Part model, mm, in its own coordinate system. Give positions to 0.01 mm unless a question says otherwise; leave off trailing zeros. Order: outer loops, then holes, each group sorted by start corner. A loop starts at its lowest first (then second) coordinate and runs counter-clockwise, first axis right, second up. Notation, with made-up numbers: M -7,-1 L 41,-1 A20 ccw 41,21 Z; hole C 74.5,-27.5 d11. An arc over 180 degrees is marked long. Return JSON: item names as keys, results as strings.
from build123d import *

# Parameters (mm, degrees)
SKETCH1_W                        = 2413
SKETCH1_H                        = 41.5544
BASE_FLANGE1_DEPTH               = 3.2639
SKETCH66_R                       = 38.1
BOSS_EXTRUDE1_DEPTH              = 3.2639
EDGE_FLANGE1_DEPTH               = 1129.41735
EDGE_FLANGE1_BEND_DEPTH          = 1066.86985
EDGE_FLANGE1_BEND_2_DEPTH        = 1066.86985
EDGE_FLANGE1_BEND_3_DEPTH        = 1129.41735
F_10_0_1935_DIAMETER_HOLE1_D     = 4.9149
F_10_0_1935_DIAMETER_HOLE1_DEPTH = 3.2649
LPATTERN1_COUNT                  = 6
LPATTERN1_PITCH                  = 215.265
F_10_0_1935_DIAMETER_HOLE2_D     = 4.9149
LPATTERN2_START                  = 22.0472
LPATTERN2_OUTLINE_R              = 2.45745
LPATTERN2_DEPTH                  = 3.2639
MIRROR1_COPY_1_D                 = 4.9149
MIRROR1_COPY_1_DEPTH             = 3.2649
MIRROR1_COPY_2_D                 = 4.9149
MIRROR1_COPY_2_DEPTH             = 3.2649
MIRROR1_COPY_3_D                 = 4.9149
MIRROR1_COPY_3_DEPTH             = 3.2649
MIRROR1_COPY_4_D                 = 4.9149
MIRROR1_COPY_4_DEPTH             = 3.2649
MIRROR1_COPY_5_D                 = 4.9149
MIRROR1_COPY_5_DEPTH             = 3.2649
F_10_0_1935_DIAMETER_HOLE4_D     = 4.9149
F_3_16_0_205_DOWEL_HOLE1_D       = 5.207
FILLET1_R                        = 25.4
FILLET2_R                        = 12.7


# Read off the part's stored shape, not the designer's step: LPattern2
# Sheet-metal steps are written as plain solids
with BuildPart() as part:
    # Sketch1 → Base-Flange1 (new body)
    with BuildSketch(Plane.XY):
        Rectangle(SKETCH1_W, SKETCH1_H)
    extrude(amount=-BASE_FLANGE1_DEPTH)

    # Sketch66 → Boss-Extrude1 (add, through all)
    with BuildSketch(Plane(origin=(0, 0, -3.2639), x_dir=(-1, 0, 0), z_dir=(0, 0, -1))):
        with Locations((-1206.5, 0)):
            Circle(SKETCH66_R)
        with Locations((1206.5, 0)):
            Circle(SKETCH66_R)
    extrude(amount=-BOSS_EXTRUDE1_DEPTH)

    # Edge-Flange1 section (across the edge) → Edge-Flange1 (add)
    with BuildSketch(Plane(origin=(-1169.9875, -22.0472, 0), x_dir=(0, 1, 0), z_dir=(1, 0, 0))):
        with BuildLine():
            Line((-3.2639, 1.27), (-3.2639, 28.4861))
            Line((-3.2639, 28.4861), (0, 28.4861))
            Line((0, 28.4861), (0, 1.27))
            ThreePointArc((0, 1.27), (0.371974388, 0.371974388), (1.27, 0))
            Line((1.27, 0), (1.27, -3.2639))
            ThreePointArc((1.27, -3.2639), (-1.935951435, -1.935951435), (-3.2639, 1.27))
        make_face()
    extrude(amount=EDGE_FLANGE1_DEPTH)

    # Edge-Flange1 section 2 (across the edge) → Edge-Flange1 bend (add)
    with BuildSketch(Plane(origin=(-40.57015, 22.0472, 0), x_dir=(0, -1, 0), z_dir=(-1, 0, 0))):
        with BuildLine():
            Line((-3.2639, 1.27), (-3.2639, 28.4861))
            Line((-3.2639, 28.4861), (0, 28.4861))
            Line((0, 28.4861), (0, 1.27))
            ThreePointArc((0, 1.27), (0.371974388, 0.371974388), (1.27, 0))
            Line((1.27, 0), (1.27, -3.2639))
            ThreePointArc((1.27, -3.2639), (-1.935951435, -1.935951435), (-3.2639, 1.27))
        make_face()
    extrude(amount=EDGE_FLANGE1_BEND_DEPTH)

    # Edge-Flange1 section 3 (across the edge) → Edge-Flange1 bend 2 (add)
    with BuildSketch(Plane(origin=(1107.44, 22.0472, 0), x_dir=(0, -1, 0), z_dir=(-1, 0, 0))):
        with BuildLine():
            Line((-3.2639, 1.27), (-3.2639, 28.4861))
            Line((-3.2639, 28.4861), (0, 28.4861))
            Line((0, 28.4861), (0, 1.27))
            ThreePointArc((0, 1.27), (0.371974388, 0.371974388), (1.27, 0))
            Line((1.27, 0), (1.27, -3.2639))
            ThreePointArc((1.27, -3.2639), (-1.935951435, -1.935951435), (-3.2639, 1.27))
        make_face()
    extrude(amount=EDGE_FLANGE1_BEND_2_DEPTH)

    # Edge-Flange1 section 4 (across the edge) → Edge-Flange1 bend 3 (add)
    with BuildSketch(Plane(origin=(40.57015, -22.0472, 0), x_dir=(0, 1, 0), z_dir=(1, 0, 0))):
        with BuildLine():
            Line((-3.2639, 1.27), (-3.2639, 28.4861))
            Line((-3.2639, 28.4861), (0, 28.4861))
            Line((0, 28.4861), (0, 1.27))
            ThreePointArc((0, 1.27), (0.371974388, 0.371974388), (1.27, 0))
            Line((1.27, 0), (1.27, -3.2639))
            ThreePointArc((1.27, -3.2639), (-1.935951435, -1.935951435), (-3.2639, 1.27))
        make_face()
    extrude(amount=EDGE_FLANGE1_BEND_3_DEPTH)

    # #10 (0.1935) Diameter Hole1
    with Locations(Plane(origin=(0, -25.3111, 0), x_dir=(-1, 0, 0), z_dir=(0, -1, 0))):
        with Locations((59.62015, -14.2875)):
            f_10_0_1935_diameter_hole1 = Hole(F_10_0_1935_DIAMETER_HOLE1_D / 2, depth=F_10_0_1935_DIAMETER_HOLE1_DEPTH)

    # LPattern1: #10 (0.1935) Diameter Hole1 ×6
    with Locations(*[(-i * LPATTERN1_PITCH, 0, 0) for i in range(1, LPATTERN1_COUNT)]):
        add(f_10_0_1935_diameter_hole1, mode=Mode.SUBTRACT)

    # #10 (0.1935) Diameter Hole2 (through all)
    with Locations(Plane(origin=(0, 25.3111, 0), x_dir=(1, 0, 0), z_dir=(0, 1, 0))):
        with Locations((-59.62015, -14.2875)):
            f_10_0_1935_diameter_hole2 = Hole(F_10_0_1935_DIAMETER_HOLE2_D / 2)

    # LPattern2 outline → LPattern2 (cut)
    with BuildSketch(Plane(origin=(0, 0, 0), x_dir=(1, 0, 0), z_dir=(0, 1, 0)).offset(LPATTERN2_START)):
        with Locations((-1074.03265, -14.2875)):
            Circle(LPATTERN2_OUTLINE_R)
        with Locations((-871.15015, -14.2875)):
            Circle(LPATTERN2_OUTLINE_R)
        with Locations((-668.26765, -14.2875)):
            Circle(LPATTERN2_OUTLINE_R)
        with Locations((-465.38515, -14.2875)):
            Circle(LPATTERN2_OUTLINE_R)
        with Locations((-262.50265, -14.2875)):
            Circle(LPATTERN2_OUTLINE_R)
    lpattern2 = extrude(amount=LPATTERN2_DEPTH, mode=Mode.SUBTRACT)

    # Mirror1: #10 (0.1935) Diameter Hole1, #10 (0.1935) Diameter Hole2, LPattern2 across plane
    add(f_10_0_1935_diameter_hole1.mirror(Plane(origin=(0, 0, 0), x_dir=(0, 0, 1), z_dir=(1, 0, 0))), mode=Mode.SUBTRACT)
    add(f_10_0_1935_diameter_hole2.mirror(Plane(origin=(0, 0, 0), x_dir=(0, 0, 1), z_dir=(1, 0, 0))), mode=Mode.SUBTRACT)
    add(lpattern2.mirror(Plane(origin=(0, 0, 0), x_dir=(0, 0, 1), z_dir=(1, 0, 0))), mode=Mode.SUBTRACT)

    # Mirror1 copy 1
    with Locations(Plane(origin=(215.265, -25.3111, 0), x_dir=(1, 0, 0), z_dir=(0, -1, 0))):
        with Locations((59.62015, 14.2875)):
            Hole(MIRROR1_COPY_1_D / 2, depth=MIRROR1_COPY_1_DEPTH)

    # Mirror1 copy 2
    with Locations(Plane(origin=(430.53, -25.3111, 0), x_dir=(1, 0, 0), z_dir=(0, -1, 0))):
        with Locations((59.62015, 14.2875)):
            Hole(MIRROR1_COPY_2_D / 2, depth=MIRROR1_COPY_2_DEPTH)

    # Mirror1 copy 3
    with Locations(Plane(origin=(645.795, -25.3111, 0), x_dir=(1, 0, 0), z_dir=(0, -1, 0))):
        with Locations((59.62015, 14.2875)):
            Hole(MIRROR1_COPY_3_D / 2, depth=MIRROR1_COPY_3_DEPTH)

    # Mirror1 copy 4
    with Locations(Plane(origin=(861.06, -25.3111, 0), x_dir=(1, 0, 0), z_dir=(0, -1, 0))):
        with Locations((59.62015, 14.2875)):
            Hole(MIRROR1_COPY_4_D / 2, depth=MIRROR1_COPY_4_DEPTH)

    # Mirror1 copy 5
    with Locations(Plane(origin=(1076.325, -25.3111, 0), x_dir=(1, 0, 0), z_dir=(0, -1, 0))):
        with Locations((59.62015, 14.2875)):
            Hole(MIRROR1_COPY_5_D / 2, depth=MIRROR1_COPY_5_DEPTH)

    # #10 (0.1935) Diameter Hole4 (through all)
    with Locations(Plane(origin=(0, 0, -3.2639), x_dir=(-1, 0, 0), z_dir=(0, 0, -1))):
        with Locations((-22.225, 12.7), (-22.225, -12.7), (22.225, -12.7), (22.225, 12.7)):
            Hole(F_10_0_1935_DIAMETER_HOLE4_D / 2)

    # 3/16 (0.205) Dowel Hole1 (through all)
    with Locations(Plane(origin=(0, 0, -3.2639), x_dir=(-1, 0, 0), z_dir=(0, 0, -1))):
        with Locations((-1208.653632912, 26.310584015), (-1184.676526013, -3.298677116), (-1214.285787144, -27.275784015), (-1238.262894043, 2.333477116)):
            f_3_16_0_205_dowel_hole1 = Hole(F_3_16_0_205_DOWEL_HOLE1_D / 2)

    # Mirror2: 3/16 (0.205) Dowel Hole1 across plane
    add(f_3_16_0_205_dowel_hole1.mirror(Plane(origin=(0, 0, 0), x_dir=(0, 0, 1), z_dir=(1, 0, 0))), mode=Mode.SUBTRACT)

    # Fillet1
    # the kernel refuses this fillet: 25.4 mm, written as the material it adds along each edge
    with BuildSketch(Plane(origin=(1174.563845564, -20.7772, 0), x_dir=(0.6276468815882087, -0.778498164437526, 0), z_dir=(0, 0, -1))) as fillet1_piece_1:
        with BuildLine():
            CenterArc((10.318975145, 25.268654931), FILLET1_R, 238.711829653, 25.458889439)
            Line((-2.872329022, 3.562676621), (-3.136155106, 3.128557055))
            ThreePointArc((-3.136155106, 3.128557055), (-1.831641579, 1.462493695), (-0.395477068, -0.318844616))
            Line((-0.395477068, -0.318844616), (0.051594876, -0.505373099))
            ThreePointArc((0.051594876, -0.505373099), (3.86961568, -0.310982396), (7.687636483, -0.505373099))
            Line((7.687636483, -0.505373099), (7.739231359, 0))
        make_face()
    extrude(amount=3.2639)
    with BuildSketch(Plane(origin=(1174.563845564, 20.7772, 0), x_dir=(0.640777338935112, 0.7677267755570576, 0), z_dir=(0, 0, -1))) as fillet1_piece_2:
        with BuildLine():
            CenterArc((12.034003451, -25.221199864), FILLET1_R, 96.802362748, 43.347829096)
            Line((-7.466256648, -8.945455455), (-7.85626185, -8.619940566))
            Line((-7.85626185, -8.619940566), (-0.390005202, 0.325514888))
            Line((-0.390005202, 0.325514888), (0.060170017, 0.504423997))
            ThreePointArc((0.060170017, 0.504423997), (4.512751294, 0.239799795), (8.965332571, 0.504423997))
            Line((8.965332571, 0.504423997), (9.025502588, 0))
        make_face()
    extrude(amount=3.2639)
    with BuildSketch(Plane(origin=(-1174.563845564, 20.7772, 0), x_dir=(1, 0, 0), z_dir=(0, 0, -1))) as fillet1_piece_3:
        with BuildLine():
            CenterArc((11.651873739, -25.4), FILLET1_R, 90, 43.347829096)
            Line((-5.783337531, -6.92912), (-6.132041757, -6.5597024))
            ThreePointArc((-6.132041757, -6.5597024), (-3.075769489, -3.310901725), (-0.425815392, 0.277029333))
            Line((-0.425815392, 0.277029333), (0, 0.508))
            Line((0, 0.508), (11.651873739, 0.508))
            Line((11.651873739, 0.508), (11.651873739, 0))
        make_face()
    extrude(amount=3.2639)
    with BuildSketch(Plane(origin=(-1174.563845564, -20.7772, 0), x_dir=(1, 0, 0), z_dir=(0, 0, -1))) as fillet1_piece_4:
        with BuildLine():
            CenterArc((13.19492891, 23.893095679), FILLET1_R, 224.706007222, 25.458889439)
            Line((-4.857504428, 6.024977407), (-5.218553095, 5.667615042))
            ThreePointArc((-5.218553095, 5.667615042), (-2.670851438, 2.817301573), (-0.425815392, -0.277029333))
            Line((-0.425815392, -0.277029333), (0, -0.508))
            ThreePointArc((0, -0.508), (2.288172782, -0.508), (4.403973897, -0.477861914))
            Line((4.403973897, -0.477861914), (4.576345564, 0))
        make_face()
    extrude(amount=3.2639)

    # Fillet2
    fillet2_edges = [part.edges().sort_by_distance(p)[0] for p in [
        (1107.44, 23.67915, 28.4861),
        (40.57015, 23.67915, 28.4861),
        (40.57015, -23.67915, 28.4861),
        (1169.9875, -23.67915, 28.4861),
        (-1169.9875, -23.67915, 28.4861),
        (-40.57015, -23.67915, 28.4861),
        (-40.57015, 23.67915, 28.4861),
        (-1107.44, 23.67915, 28.4861),
    ]]
    fillet(fillet2_edges, radius=FILLET2_R)


solid = part.part
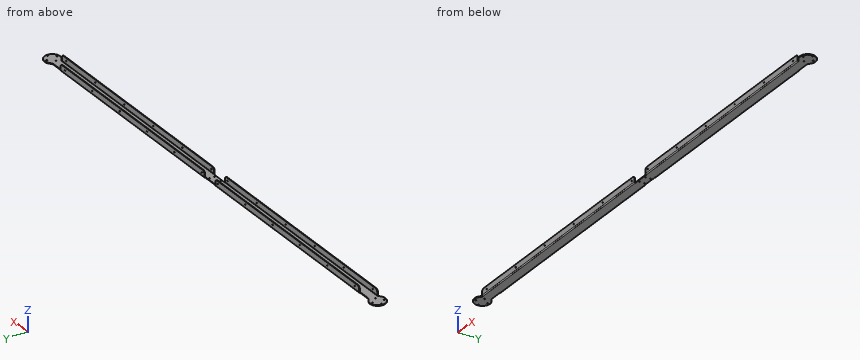
Q1. Band-saw the part on B-B (x = 310). Give the cut face in (y, z).
Established:
{"outline": "M -25.31,1.27 A4.53 ccw -20.78,-3.26 L 20.78,-3.26 A4.53 ccw 25.31,1.27 L 25.31,28.49 L 22.05,28.49 L 22.05,1.27 A1.27 cw 20.78,0 L -20.78,0 A1.27 cw -22.05,1.27 L -22.05,28.49 L -25.31,28.49 Z"}
Q2. Band-saw the part on A-A (z = 23.5). Give the cut face in (x, y), then the cut area to 3 significant figures.
Established:
{"outline": "M -1167.38,-25.31 L -43.18,-25.31 L -43.18,-22.05 L -1167.38,-22.05 Z; M -1104.83,22.05 L -43.18,22.05 L -43.18,25.31 L -1104.83,25.31 Z; M 43.18,-25.31 L 1167.38,-25.31 L 1167.38,-22.05 L 43.18,-22.05 Z; M 43.18,22.05 L 1104.83,22.05 L 1104.83,25.31 L 43.18,25.31 Z", "area": "14,300 mm²"}
Q3. Pin check, flat tips, straight feed: pin 1 (3 mm diameter, centred on x = 690, y = 6, fed in from +Z); pin 2 (3 mm diameter, centred on x = 1184.68, y = -3.3, fed in from +Z); pin 3 (5.5 mm diameter, centred on x = -262.5, z = 14.29, fed in from +Y); pin 4 (13.5 mm diameter, centred on x = 512.5, z = 10, fed in from -Y). Stop position of each tip, or through.
Established:
{"pin 1": "stops at z = 0", "pin 2": "passes through", "pin 3": "stops at y = 25.31", "pin 4": "stops at y = -25.31"}
Q4. Probe line 1 along Y through (x, z) = (-550, 17); line 2 along X through (y, z) = (22.5, 3); line 3 along Z through (x, y) = (-689, -8). List the from-to ranges inside material, lowest first.
Established:
{"line 1": "y = -25.31 to -22.05, 22.05 to 25.31", "line 2": "x = -1107.44 to -40.57, 40.57 to 1107.44", "line 3": "z = -3.26 to 0"}
